Can you work these out from the model? Positions are in its coordinate system, mm. A direction names the side the tool comes from. Give positions to 0.01 mm unless a question says otherwise; leave off trailing zeros. Order: outer loops, then holes, each group sorted by start corner. A loop starts at its lowest first (then second) coordinate and runs counter-clockwise, first axis right, second up. Notation, with made-up numbers: (-24.75, 36) - (6.25, 36) arc R23 ccw to (6.25, 64) - close; hole circle Ø4 at (12, 78). An arc over 180 degrees is marked (long way). Answer as CSV lines item,"result".
```python
from build123d import *

# Parameters (mm, degrees)
F0_W      = 16
F0_H      = 11
F1_DEPTH  = 5
F2_W      = 2.5
F2_H      = 2.5
F2_W_2    = 3
F2_H_2    = 3
F2_W_3    = 2
F3_DEPTH  = 2
F5_FACE_W = 32
F5_FACE_H = 22
F6_DEPTH  = 3.8


with BuildPart() as f1:
    # F0 (on Top) → F1 (new body)
    with BuildSketch(Plane.XY):
        with Locations((-8, 5.5)):
            Rectangle(F0_W, F0_H)
    extrude(amount=F1_DEPTH)

    # F2 (on face) → F3 (join)
    with BuildSketch(Plane.XY.offset(5)):
        with Locations((-14.75, 9.75)):
            Rectangle(F2_W, F2_H)
        with Locations((-12, 9.75)):
            Rectangle(F2_W_2, F2_H)
        with Locations((-14.75, 7)):
            Rectangle(F2_W, F2_H_2)
        with Locations((-1, 9.75)):
            Rectangle(F2_W_3, F2_H)
    extrude(amount=F3_DEPTH)

    # F4: F1 across plane


with BuildPart() as f1_1:
    add(f1.part)
    add(f1.part.mirror(Plane.XZ))

    # F5: F1 across plane


with BuildPart() as f1_2:
    add(f1_1.part)
    add(f1_1.part.mirror(Plane.YZ))

    # F5_face (on face) → F6 (join)
    with BuildSketch(Plane(origin=(0, 0, 0), x_dir=(1, 0, 0), z_dir=(0, 0, -1))):
        Rectangle(F5_FACE_W, F5_FACE_H)
    extrude(amount=F6_DEPTH)


solid = f1_2.part
```
1) I need wall thicknesses on line 1 along Y through (x, z) = (-0.5, 5.5); line 2 along Z through (x, y) = (-9, -6.75). Which ranges of each line are inside material? Lowest first, please. Write a range as [from, to].
Answer block:
line 1,"[-11, -8.5], [8.5, 11]"
line 2,"[-3.8, 5]"
2) If we mould it in two halves opening along Y, with no side actions, what happens to faces 4 (the flat face through (13.5, 7, 6)), 5 (the flat face through (0, 11, 2)), 6 (the flat face through (10.5, 10, 6)), 7 (the flat face through (0, -11, 2))? For each: +Y half, -Y half, draft (parallel to the pull), parting line (faces both ways), or undercut.
Answer block:
face 4,"undercut"
face 5,"+Y half"
face 6,"draft"
face 7,"-Y half"
3) I want a section at B-B on y = 6.25. Write out the boundary of the cut face in (x, z), plus the area to 3 significant figures.
Answer block:
outline,"(-16, -3.8) - (16, -3.8) - (16, 7) - (13.5, 7) - (13.5, 5) - (-13.5, 5) - (-13.5, 7) - (-16, 7) - close"
area,"292 mm2"
4) Which directions (+Z, -Z, +X, -X, +Y, -Y) give clear straight access to the entire face, cutting with the end or side of a thin tool? Please do faces 1 (the flat face through (-2, 10, 6)), 2 (the flat face through (-13.5, 7, 6)), 3 (the flat face through (-15, 5.5, 6)).
Answer block:
face 1,"+Z, +Y, -Y"
face 2,"+Z"
face 3,"+Z, +X, -X"
5) I want a section at A-A on z = 5.5. Count the separate pieces of the cut face and the enclosed holes in it, plus the area to 3 significant figures.
Answer block:
separate pieces,"6"
enclosed holes,"0"
area,"105 mm2"
6) I'm going to push a flat-ended pin straight in: P1, Ø3, axis at x = -8, y = 1, coming from the +Z side. Where does the tip first touch, or does it pass through?
Answer block:
P1,"z = 5"
7) I want a section at C-C on x = -1. Write out the boundary of the cut face in (y, z), plus the area to 3 significant figures.
Answer block:
outline,"(-11, -3.8) - (11, -3.8) - (11, 7) - (8.5, 7) - (8.5, 5) - (-8.5, 5) - (-8.5, 7) - (-11, 7) - close"
area,"204 mm2"
